Can you work these out from the model? Positions are in its coordinate system, mm. Face numbers are marked on the shaded views. Give positions to 0.01 mm unless a question says otherwise; leave off trailing zeros. Order: outer loops, then holes, each group sorted by start corner. A loop starts at its lowest first (then second) coordinate and runs counter-clockwise, first axis right, second up.
Item 1: If we mould it in two halves opening along Z, with no side actions, what happens to the marked faces 1, 2, 3 and 4? For each: +Z half, -Z half, draft (parallel to the pull), parting line (faces both ways), or undercut.
Item 2: I want a section at C-C, the plane y = -84. Write out the boundary of the cut face in (x, z) (3 decimals).
Item 3: I want a section at B-B, the plane x = 17.5. Write out the boundary of the cut face in (y, z) (3 decimals).
Item 4: I'm going to push a flat-ended pin straight in: pin 1 Ø8 at (x, z) = (-6, -7.5) entering from +Y. Where does the tip first touch, or does it pass through?
Item 5: I want a section at A-A, the plane z = 6. Write out the boundary of the cut face in (x, y) (3 decimals), then the cut area to 3 significant figures.
Item 6: If I drill on line 1 along X through (y, z) = (25.5, 3) (3 decimals); line 2 along Z through (x, y) = (2, 102) (3 decimals); line 3 along X through (y, z) = (122, 4) (3 decimals), over which ranges is the centre line in solid material (lowest first)?
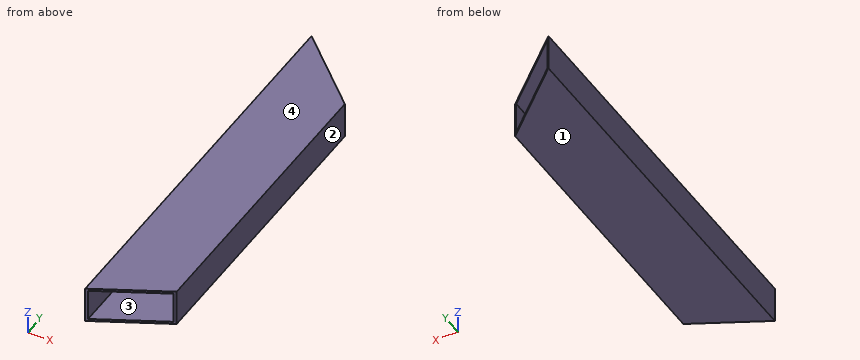
```python
from build123d import *

# Parameters (mm, degrees)
F0_W        = 50
F0_H        = 25
F0_W_2      = 46.83
F0_H_2      = 21.83
F1_DEPTH    = 141.91
F2_T1_DEPTH = 288.1699043199
F3_T1_DEPTH = 286.404275023


# Not quite as in the source:
# - a fillet or chamfer that OpenCascade refuses, or shapes differently, is made with other operations: its cross-section is extruded or revolved along the edge and cut away or added


with BuildPart() as f1:
    # F0 (on Front) → F1 (new body, symmetric)
    with BuildSketch(Plane.XZ):
        Rectangle(F0_W, F0_H)
        Rectangle(F0_W_2, F0_H_2, mode=Mode.SUBTRACT)
    extrude(amount=F1_DEPTH, both=True)

    # F2: chamfer of 50.8 x 24.77 on 1 edges, made by hand

    # F2_s2 → F2_t1 (cut)
    with BuildSketch(Plane.XY.offset(-144.08495216)):
        Polygon((25, -117.14), (-25.8, -141.91), (25, -141.91), align=None)
    extrude(amount=F2_T1_DEPTH, mode=Mode.SUBTRACT)

    # F3: chamfer of 50.8 x 49.05 on 1 edges, made by hand

    # F3_s2 → F3_t1 (cut)
    with BuildSketch(Plane.XY.offset(-143.2021375115)):
        Polygon((-25.8, 141.91), (25, 92.86), (25, 141.91), align=None)
    extrude(amount=F3_T1_DEPTH, mode=Mode.SUBTRACT)


solid = f1.part
```
Results list:
1. face 1: -Z half
1. face 2: draft
1. face 3: undercut
1. face 4: +Z half
2. outline: (-25, -12.5) - (25, -12.5) - (25, 12.5) - (-25, 12.5) - close; hole (-23.415, -10.915) - (23.415, -10.915) - (23.415, 10.915) - (-23.415, 10.915) - close
3. outline: (-120.797, -12.5) - (100.102, -12.5) - (100.102, -10.915) - (-120.797, -10.915) - close; (-120.797, 10.915) - (100.102, 10.915) - (100.102, 12.5) - (-120.797, 12.5) - close
4. pin 1: stops at y = 124.8
5. outline: (-25, -141.52) - (-23.415, -140.747) - (-23.415, 139.607) - (-25, 141.138) - close; (23.415, -117.913) - (25, -117.14) - (25, 92.86) - (23.415, 94.39) - close
5. area: 781 mm2
6. line 1: x = -25 to -23.415, 23.415 to 25
6. line 2: z = -12.5 to -10.915, 10.915 to 12.5
6. line 3: x = -25 to -23.415
